Check sheet for the drawn part. Datum: minimum x, y, z corner. Units: mm. A direction names the side the tool comes from. Coordinates: 2 decimals unless noted, no trailing zeros. Loops run counter-clockwise (first coordinate to the right, second up) from the corner with the lowest first, then second, coordinate; pieces in that order, holes last. Notation, with made-up numbers: M 37,-1.5 L 89,-1.5 A19 ccw 89,20.5 Z; hole C 7,-25.5 d1. An arc over 180 degrees is marked long. Answer in a Markdown table with one row per item. Add a question column.
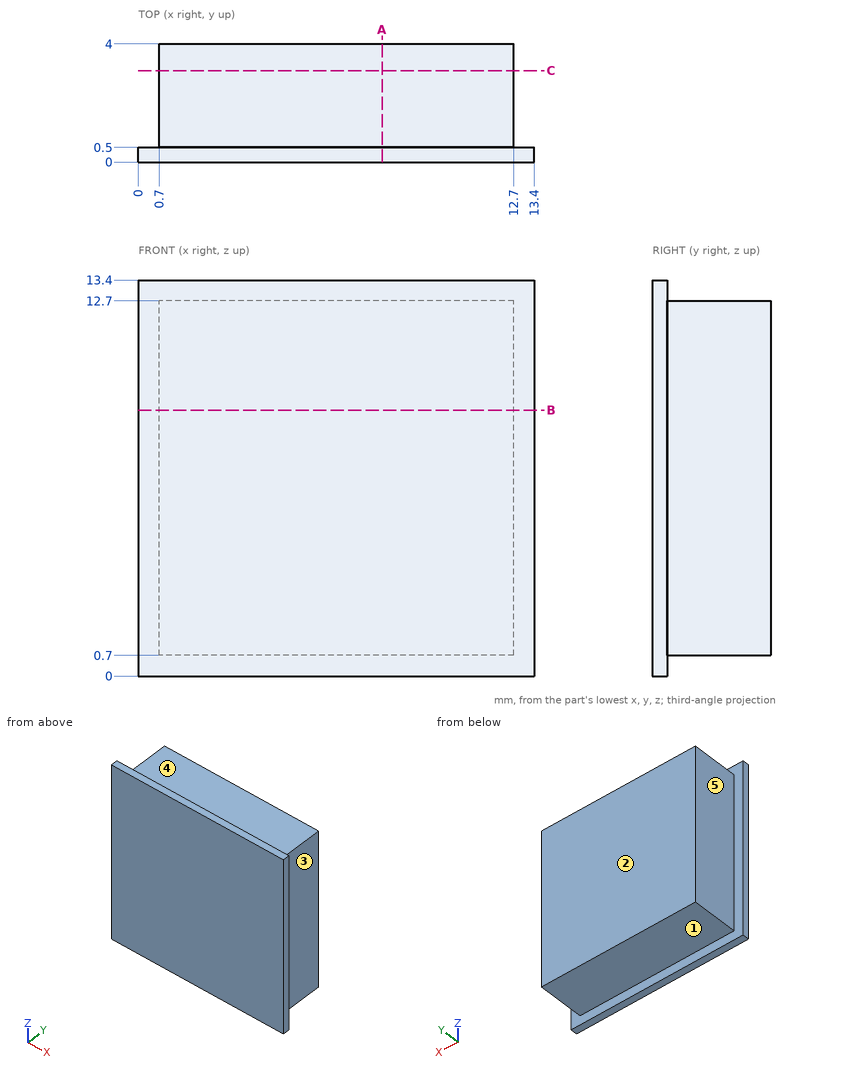
Q1. Cross-section at A-A (x = 8.25). Record the cut outline in (y, z).
Q2. Access from +Z, -Z, +X, -X, +Y, -Y to the whole of each face (thin tool, end or side, straight path). Record for the marked faces 1 and 2.
Q3. Mould release check, pull along X, two halves, no side actions. Record for the marked faces 3, 4 and 5: released by +X, released by -X, zero draft, split by the parting line, or undercut.
Q4. Thickness scan on L1, parallel to X at y = 3.25, z = 7; L2, parallel to Y at x = 11.75, z = 0.5. Record the ranges inside material, lowest first.
Q5. Cross-section at B-B (z = 9). Record the cut outline in (x, y).
Q6. Go/stop test with flat-tipped pins: pin 1 (1 mm diameter, centred on x = 8.5, y = 2, fed in from -Z); pin 2 (1 mm diameter, centred on y = 2.5, z = 7.5, fed in from +X); pin 3 (1.8 mm diameter, centred on x = 6.5, y = 2, fed in from +Z). Record where each tip stops, or that it passes through.
Q7. Cross-section at C-C (y = 3.1). Record the cut outline in (x, z), plus the area to 3 significant figures.
Answer key:
| question | item | result |
|---|---|---|
| 1 | outline | M 0,0 L 0.5,0 L 0.5,0.7 L 4,0.7 L 4,12.7 L 0.5,12.7 L 0.5,13.4 L 0,13.4 Z |
| 2 | face 1 | -Z, +X, -X, +Y |
| 2 | face 2 | +Z, -Z, +X, -X, +Y |
| 3 | face 3 | released by +X |
| 3 | face 4 | zero draft |
| 3 | face 5 | released by -X |
| 4 | L1 | 0.7 to 12.7 |
| 4 | L2 | 0 to 0.5 |
| 5 | outline | M 0,0 L 13.4,0 L 13.4,0.5 L 12.7,0.5 L 12.7,4 L 0.7,4 L 0.7,0.5 L 0,0.5 Z |
| 6 | pin 1 | z = 0.7 |
| 6 | pin 2 | x = 12.7 |
| 6 | pin 3 | z = 12.7 |
| 7 | outline | M 0.7,0.7 L 12.7,0.7 L 12.7,12.7 L 0.7,12.7 Z |
| 7 | area | 144 mm^2 |
